Autodesk Inventor part; units mm, degrees
ref_plane "YZ Plane" through (0, 0, 0) normal (1, 0, 0) x (0, 1, 0)
ref_plane "XZ Plane" through (0, 0, 0) normal (0, 1, 0) x (-1, 0, 0)
ref_plane "XY Plane" through (0, 0, 0) normal (0, 0, 1) x (1, 0, 0)
sketch "Esquisse1" plane through (0, 0, 0) normal (1, 0, 0) x (0, 1, 0)
  line L0 (15, 8.5) -> (-15, 8.5)
  line L1 (-15, 8.5) -> (-15, -8.5)
  line L2 (-15, -8.5) -> (15, -8.5)
  line L3 (15, -8.5) -> (15, 8.5)
  point P0 (0, 0)
  point P1 (0, 0)
  point P2 (0, 0)
  dimension "d4" = 30
  dimension "d5" = 17
extrude "Extrusion1" add sketch "Esquisse1" along normal blind 10
sketch "Esquisse2" plane through (10, 0, 0) normal (1, 0, 0) x (0, 0, -1)
  line L0 (-7.5, 13.5) -> (7.5, 13.5)
  line L1 (7.5, 13.5) -> (7.5, -13.5)
  line L2 (7.5, -13.5) -> (-7.5, -13.5)
  line L3 (-7.5, -13.5) -> (-7.5, 13.5)
  line L4 (-7.5, 13.5) -> (7.5, -13.5)
  line L5 (-7.5, -13.5) -> (7.5, 13.5)
  point P0 (0, 0)
  point P1 (0, 0)
  point P2 (0, 0)
  dimension "d8" = 27
  dimension "d9" = 15
extrude "Extrusion2" cut sketch "Esquisse2" against normal blind 9
sketch "Esquisse3" plane through (1, 0, 0) normal (1, 0, 0) x (0, 0, -1)
  line L0 (7.5, -13.5) -> (-7.5, -13.5)
  line L1 (7.5, 13.5) -> (7.5, -13.5)
  line L2 (-7.5, -13.5) -> (7.5, -13.5)
  line L3 (7.5, -13.5) -> (7.5, -7.5)
  line L4 (7.5, -7.5) -> (-7.5, -7.5)
  line L5 (-7.5, -7.5) -> (-7.5, -13.5)
  point P0 (0, 0)
  dimension "d12" = 6
extrude "Extrusion3" cut sketch "Esquisse3" against normal blind 9
sketch "Esquisse4" plane through (0, 15, 8.5) normal (0, 1, 0) x (1, 0, 0)
  line L0 (0, 0) -> (0, 17)
  line L1 (0, 0) -> (10, 0)
  line L2 (0, 17) -> (3, 17)
  line L3 (3, 17) -> (3, 0)
  line L4 (3, 0) -> (0, 0)
  line L5 (0, 0) -> (0, 17)
  point P0 (0, 8.5)
extrude "Extrusion4" add sketch "Esquisse4" along normal blind 9
sketch "Esquisse5" plane through (3, 15, 8.5) normal (1, 0, 0) x (0, 0, -1)
  circle A0 centre (13.5, 5) radius 1.75
  line L0 (17, 9) -> (0, 9)
  line L1 (8.5, 9) -> (8.5, 0)
  line L2 (17, 0) -> (0, 0)
  circle A1 centre (3.5, 5) radius 1.75
  point P0 (8.5, -15)
  dimension "d17" = 3.5
  dimension "d18" = 5
  dimension "d19" = 4
extrude "Extrusion5" cut sketch "Esquisse5" against normal blind 3
fillet "Congé1" radius 2 2 edges at (1.5, 24, -8.5) (1.5, 24, 8.5)
fillet "Congé2" radius 1.5 2 edges at (5, -15, 8.5) (5, -15, -8.5)
properties part number "support_tof_actionneur_panneaux_solaires_Impression 3D"
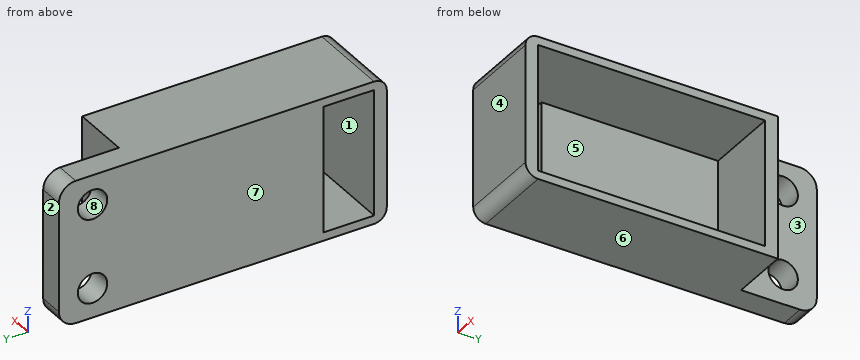
Check sheet for the modelled part. Datum: model origin and axes. Units: mm. Face numbers are marked on the shaded views. A direction names the side the tool comes from. Round coordinates to 2 decimals unless told otherwise and drop trailing zeros. Order: outer loops, then holes, each group sorted by start corner. A loop starts at its lowest first (then second) coordinate and runs counter-clockwise, first axis right, second up. Notation, with made-up numbers: (-7.75, 69) - (20.25, 69) arc R27 cw to (20.25, 104) - close; hole circle Ø7 at (11, 2). An arc over 180 degrees is marked (long way). Write item = value, one per line.
Q1. Section check C-C (z = -1.25). Record the boundary of the cut face in (x, y).
Computed:
outline = (0, -15) - (10, -15) - (10, -13.5) - (0, -13.5) - close; (0, -7.5) - (1, -7.5) - (1, 13.5) - (10, 13.5) - (10, 15) - (3, 15) - (3, 24) - (0, 24) - close
Q2. Section check D-D (x = 0.5). Record the boundary of the cut face in (y, z).
Computed:
outline = (-15, -7) arc R1.5 ccw to (-13.5, -8.5) - (22, -8.5) arc R2 ccw to (24, -6.5) - (24, 6.5) arc R2 ccw to (22, 8.5) - (-13.5, 8.5) arc R1.5 ccw to (-15, 7) - close; hole (-13.5, -7.5) - (-7.5, -7.5) - (-7.5, 7.5) - (-13.5, 7.5) - close; hole circle Ø3.5 at (20, -5); hole circle Ø3.5 at (20, 5)
Q3. Tool access check on the marked faces 1, 2, 3, 4 and 5. Record the directions out of +Z, -Z, +X, -X, +Y, -Y that give a thin tool (end or side, any length) a straight path to the whole face; none if there is none.
Computed:
face_1 = +X, -X
face_2 = +Z, -Z, +X, -X, +Y
face_3 = +Z, -Z, +X, +Y
face_4 = +Z, -Z, +X, -X, -Y
face_5 = +X
Q4. Section check A-A (z = -5). Record the boundary of the cut face in (x, y), and give its area (3 significant figures).
Computed:
outline = (0, -15) - (10, -15) - (10, -13.5) - (0, -13.5) - close; (0, -7.5) - (1, -7.5) - (1, 13.5) - (10, 13.5) - (10, 15) - (3, 15) - (3, 18.25) - (0, 18.25) - close; (0, 21.75) - (3, 21.75) - (3, 24) - (0, 24) - close
area = 67.5 mm^2
Q5. Thickness scan on line 1 along Y through (x, z) = (1.95, -5); line 2 along Y through (x, z) = (0.75, 5); line 3 along Y through (x, z) = (5.5, 4.5). Record the ranges inside material, lowest first.
Computed:
line_1 = -15 to -13.5, 13.5 to 18.25, 21.75 to 24
line_2 = -15 to -13.5, -7.5 to 18.25, 21.75 to 24
line_3 = -15 to -13.5, 13.5 to 15
Q6. Section check B-B (y = -10). Record the boundary of the cut face in (x, z), and give its area (3 significant figures).
Computed:
outline = (0, -8.5) - (10, -8.5) - (10, -7.5) - (0, -7.5) - close; (0, 7.5) - (10, 7.5) - (10, 8.5) - (0, 8.5) - close
area = 20.0 mm^2
Q7. Draft check along Z on the marked faces 6, 7 and 8. Enter one of: pulls with the +Z half, pulls with the -Z half, needs draft (parallel to the pull), parting line crosses it, or undercut.
Computed:
face_6 = pulls with the -Z half
face_7 = needs draft
face_8 = undercut
Q8. Go/stop test with flat-tipped pins: pin 1 (5.5 mm diameter, centred on x = 7.5, z = -2.5, fed in from +Y); pin 2 (4 mm diameter, centred on y = 20, z = 5, fed in from -X); pin 3 (4.5 mm diameter, centred on y = 3.5, z = -3, fed in from +X); pin 4 (7 mm diameter, centred on y = 20.5, z = 1.5, fed in from +X). Record where each tip stops, or that it passes through.
Computed:
pin_1 = 15
pin_2 = 0
pin_3 = 1
pin_4 = 3
